Read the model definition and answer for the solid it produces. Units are mm, in the model's axes. Face numbers are marked on the shaded views. Coordinates: 2 decimals unless noted, no trailing zeros. Loops run counter-clockwise (first coordinate to the right, second up) from the corner with the lowest first, then second, coordinate; pieces in that order, holes last. Notation, with made-up numbers: (55, -12) - (95, -12) arc R15 ccw to (95, -6) - close; hole circle Ø9 at (77, 52.5). An arc over 180 degrees is marked (long way). Use one line per item in the form item = value. Start each with the question number.
1) Each of these flat-tipped pins is pushed along its axis until it touches: P1, Ø1.5, axis at x = 14.5, y = 4, coming from the -Z side; P2, Ø6.5, axis at x = 0, z = 0, coming from the +Y side; P3, Ø12, axis at y = 7.5, z = -22.5, coming from the +X side. Where does it stop, or does it pass through?
2) A cutting plane is placed at D-D (y = 23.25). Give the vertices of the cut face in (x, z).
3) A cutting plane is placed at A-A (x = 0). Give the vertices of the cut face in (y, z), and give its area (3 significant figures).
4) The mould has two halves that part along X. Classify the marked faces 1, 2, 3 and 4: released by +X, released by -X, zero draft, split by the parting line, or undercut.
5) Consider line 1 (Z direction, x = 0, y = 16.5); line 2 (Z direction, x = 0, y = 1.9). Determine where each line is inside the solid, lowest interval first.
6) A cutting plane is placed at B-B (z = 0). Give the vertices of the cut face in (x, y).
7) A cutting plane is placed at C-C (y = 13.25). Give the vertices of the cut face in (x, z).
from build123d import *

# Parameters (mm, degrees)
SKETCH1_R               = 37.75
BOSS_EXTRUDE1_DEPTH     = 5
SKETCH2_R               = 37.75
SKETCH2_R_2             = 31.7505
BOSS_EXTRUDE2_DEPTH     = 20
CHAMFER1_SIZE           = 5
CHAMFER1_SIZE2          = 4.195498156
SKETCH3_R               = 2.55
CUT_EXTRUDE1_DEPTH      = 1
CUT_EXTRUDE1_DEPTH_BACK = 26


with BuildPart() as part:
    # Sketch1 → Boss-Extrude1 (new body)
    with BuildSketch(Plane(origin=(0, 0, 0), x_dir=(1, 0, 0), z_dir=(0, 1, 0))):
        Circle(SKETCH1_R)
    extrude(amount=BOSS_EXTRUDE1_DEPTH)

    # Sketch2 → Boss-Extrude2 (add)
    with BuildSketch(Plane(origin=(0, 5, 0), x_dir=(1, 0, 0), z_dir=(0, 1, 0))):
        Circle(SKETCH2_R)
        Circle(SKETCH2_R_2, mode=Mode.SUBTRACT)
    extrude(amount=BOSS_EXTRUDE2_DEPTH)

    # Chamfer1
    chamfer1_edges = [part.edges().sort_by_distance(p)[0] for p in [
        (-37.75, 25, 0),
    ]]
    chamfer1_side = [part.faces().sort_by_distance(p)[0] for p in [
        (-37.75, 12.5, 0),
    ]]
    chamfer(chamfer1_edges, length=CHAMFER1_SIZE, length2=CHAMFER1_SIZE2, reference=chamfer1_side[0])

    # Sketch3 → Cut-Extrude1 (cut, two sides)
    with BuildSketch(Plane.XZ) as cut_extrude1_sk:
        Circle(SKETCH3_R)
    extrude(amount=CUT_EXTRUDE1_DEPTH, mode=Mode.SUBTRACT)
    extrude(cut_extrude1_sk.sketch, amount=-CUT_EXTRUDE1_DEPTH_BACK, mode=Mode.SUBTRACT)


solid = part.part
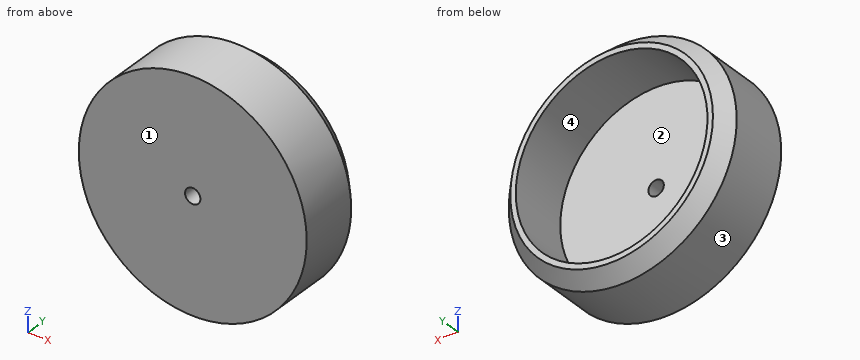
Found:
q1.P1 = -35.16
q1.P2 = 5
q1.P3 = 33.95
q2.outline = circle Ø70.05 at (0, 0); hole circle Ø63.5 at (0, 0)
q3.outline = (0, -37.75) - (20, -37.75) - (25, -33.55) - (25, -31.75) - (5, -31.75) - (5, -2.55) - (0, -2.55) - close; (0, 2.55) - (5, 2.55) - (5, 31.75) - (25, 31.75) - (25, 33.55) - (20, 37.75) - (0, 37.75) - close
q3.area = 571 mm^2
q4.face_1 = zero draft
q4.face_2 = undercut
q4.face_3 = split by the parting line
q4.face_4 = undercut
q5.line_1 = -37.75 to -31.75, 31.75 to 37.75
q5.line_2 = -37.75 to -2.55, 2.55 to 37.75
q6.outline = (-37.75, 0) - (-2.55, 0) - (-2.55, 5) - (-31.75, 5) - (-31.75, 25) - (-33.55, 25) - (-37.75, 20) - close; (2.55, 0) - (37.75, 0) - (37.75, 20) - (33.55, 25) - (31.75, 25) - (31.75, 5) - (2.55, 5) - close
q7.outline = circle Ø75.5 at (0, 0); hole circle Ø63.5 at (0, 0)
